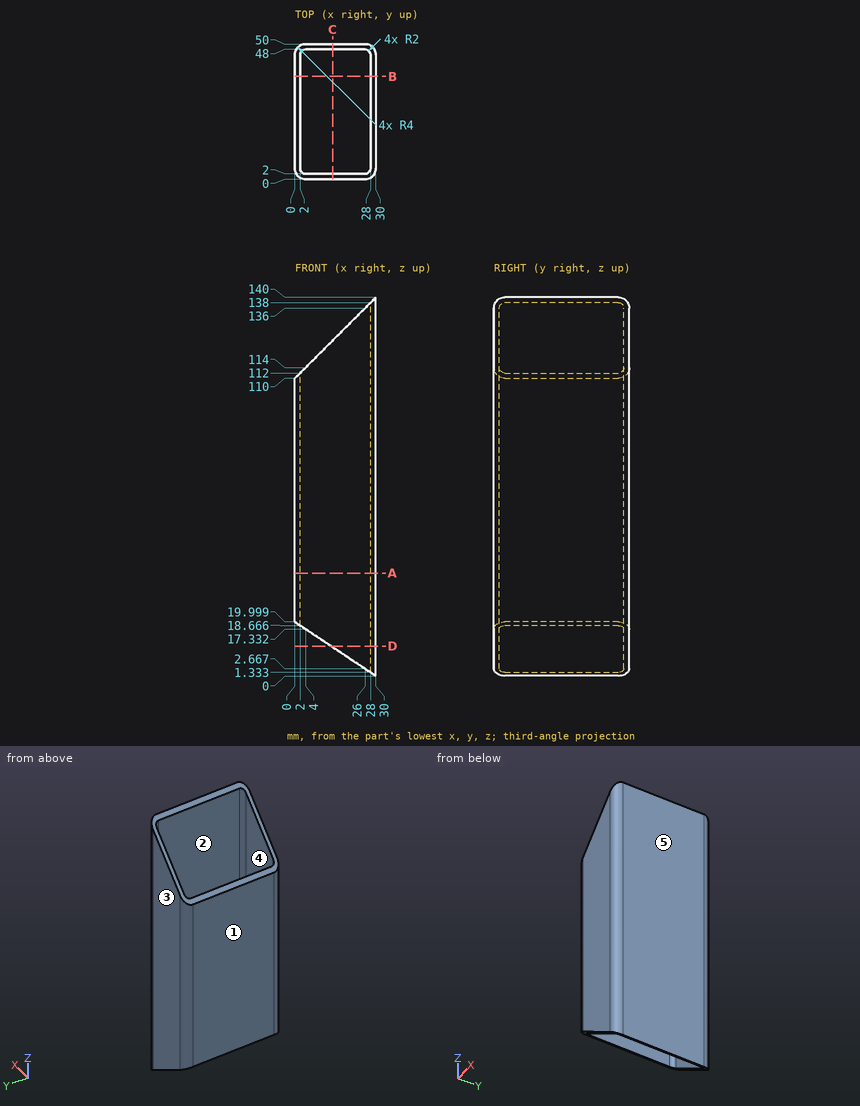
Geometry: see drawing. Coordinates: mm, zero at the bounding-box minimum. A direction names the side the tool comes from. Coordinates: 2 decimals unless noted, no trailing zeros. Write each loop counter-clockwise with the first axis right and the second up, starting at its lowest first coordinate (ties: lowest second). Pieces come first, ordered by that corner, then holes. Notation, with made-up numbers: M 0,88 L 53,88 A10 cw 53,94 Z; hole C 76.25,47 d5. An arc over 180 degrees is marked long. Use CSV: the item, a comma, the result in double quotes. Start each with the question number.
1. Cut plane B-B on y = 38. Return the cut outline in (x, z) (1 decimal).
2. Reachability of the marked faces 4 and 5 from +Z, -Z, +X, -X, +Y, -Y: full face, straight path, thin tool, end or side. Return the list, or none.
3. Ray query, probe 1 along X at (y, z) = (20, 38); probe 2 along Y at (x, z) = (14, 113); probe 3 along X at (y, z) = (21, 116.5). Return the intervals inside material, ascending.
4. First-contact query: P1, Ø2, axis at y = 44.5, z = 116.5, coming from the -X side. Flat tip, straight axial feed; report the tip coordinate or a pass-through.
5. Cut plane A-A on z = 38. Return the cut outline in (x, y).
6. Cut plane D-D on z = 11. Return the cut outline in (x, y), plus the area to 3 significant figures.
7. Cut plane C-C on x = 14. Return the cut outline in (y, z).
8. Mould query, pull axis Y, two halves, no side actions, for the marked faces 1, 2 and 3. Classes: pulls with the +Y half, pulls with the -Y half, needs draft (parallel to the pull), parting line crosses it, or undercut.
Entries:
1,outline,"M 0,20 L 2,18.7 L 2,112 L 0,110 Z; M 28,1.3 L 30,0 L 30,140 L 28,138 Z"
2,face 4,"+Z, -Z"
2,face 5,"+Z, -Z, +X, +Y, -Y"
3,probe 1,"0 to 2, 28 to 30"
3,probe 2,"0 to 2, 48 to 50"
3,probe 3,"28 to 30"
4,P1,"x = 28"
5,outline,"M 0,4 A4 ccw 4,0 L 26,0 A4 ccw 30,4 L 30,46 A4 ccw 26,50 L 4,50 A4 ccw 0,46 Z; hole M 2,4 A2 ccw 4,2 L 26,2 A2 ccw 28,4 L 28,46 A2 ccw 26,48 L 4,48 A2 ccw 2,46 Z"
6,outline,"M 13.5,0 L 26,0 A4 ccw 30,4 L 30,46 A4 ccw 26,50 L 13.5,50 L 13.5,48 L 26,48 A2 cw 28,46 L 28,4 A2 cw 26,2 L 13.5,2 Z"
6,area,"153 mm²"
7,outline,"M 0,10.67 L 2,10.67 L 2,124 L 0,124 Z; M 48,10.67 L 50,10.67 L 50,124 L 48,124 Z"
8,face 1,"needs draft"
8,face 2,"undercut"
8,face 3,"pulls with the +Y half"
